Autodesk Inventor part; units mm, degrees
ref_plane "YZ Plane" through (0, 0, 0) normal (1, 0, 0) x (0, 1, 0)
ref_plane "XZ Plane" through (0, 0, 0) normal (0, 1, 0) x (-1, 0, 0)
ref_plane "XY Plane" through (0, 0, 0) normal (0, 0, 1) x (1, 0, 0)
sketch "Sketch1" plane through (0, 0, 0) normal (0, 0, 1) x (1, 0, 0)
  line L0 (0, 0) -> (0, -25.4)
  line L1 (0, 0) -> (34.925, 0)
  line L2 (0, -25.4) -> (6.35, -25.4)
  line L3 (34.925, 0) -> (34.925, -6.35)
  line L4 (34.925, -6.35) -> (9.525, -6.35)
  line L5 (6.35, -9.525) -> (6.35, -25.4)
  arc A0 (9.525, -6.35) -> (6.35, -9.525) centre (9.525, -9.525) ccw
  dimension "d0" = 25.4
  dimension "d1" = 34.925
  dimension "d2" = 6.35
  dimension "d3" = 6.35
  dimension "d4" = 3.175
extrude "Extrusion1" add sketch "Sketch1" along normal blind 308.483
equation "\"d2\" = d3"
properties part number "Y_shaft_support_cross_bar" material "Aluminum 6061"
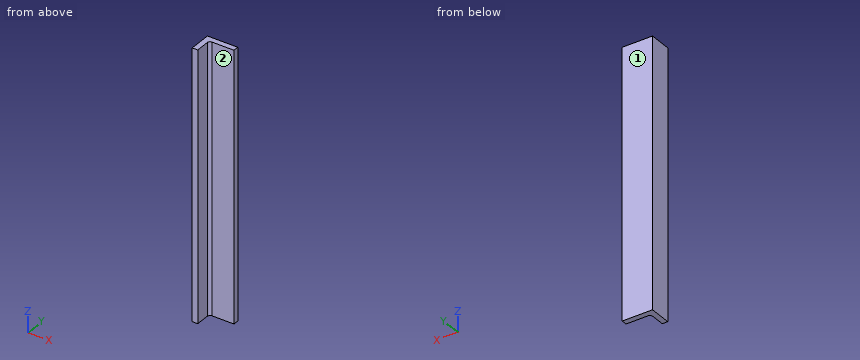
Could you check a few things on this model? Use its own coordinates, in mm. Face numbers are marked on the shaded views. A direction names the side the tool comes from. Give positions to 0.01 mm unless a question says otherwise; leave off trailing zeros. Order: outer loops, then holes, each group sorted by start corner. A loop starts at its lowest first (then second) coordinate and runs counter-clockwise, first axis right, second up.
Item 1: If we section it at A-A, the plane z = 82.5: Write out the boundary of the cut face in (x, y) (3 decimals), plus the area to 3 significant figures.
Item 2: For the marked faces 1 and 2, which set-ups out of +Z, -Z, +X, -X, +Y, -Y let a thin tool reach every point of the face, with its end or its side?
Item 3: If we section it at B-B, the plane x = 24: Write out the boundary of the cut face in (y, z).
Item 4: I need wall thicknesses on line 1 (X direction, y = -23.75, z = 56); line 2 (Y direction, x = 33, z = 272); line 3 (X direction, y = -7, z = 114.5). Which ranges of each line are inside material? Lowest first, please.
Item 5: I'm going to push flat-ended pins straight in: pin 1 (12.5 mm diameter, centred on y = -16.5, z = 186.5, fed in from +X); pin 2 (7.5 mm diameter, centred on x = 25.5, z = 153, fed in from -Y); pin 3 (6 mm diameter, centred on y = -10, z = 55.5, fed in from +X). Where does each tip first touch, or does it pass through?
Item 6: If we section it at C-C, the plane y = -14: Write out the boundary of the cut face in (x, z), plus the area to 3 significant figures.
Values:
1. outline: (0, -25.4) - (6.35, -25.4) - (6.35, -9.525) arc R3.175 cw to (9.525, -6.35) - (34.925, -6.35) - (34.925, 0) - (0, 0) - close
1. area: 345 mm2
2. face 1: +Z, -Z, +X, -X, +Y
2. face 2: +Z, -Z, +X, -Y
3. outline: (-6.35, 0) - (0, 0) - (0, 308.48) - (-6.35, 308.48) - close
4. line 1: x = 0 to 6.35
4. line 2: y = -6.35 to 0
4. line 3: x = 0 to 7.6
5. pin 1: stops at x = 6.35
5. pin 2: stops at y = -6.35
5. pin 3: stops at x = 7.6
6. outline: (0, 0) - (6.35, 0) - (6.35, 308.48) - (0, 308.48) - close
6. area: 1,960 mm2
